```python
from build123d import *

# Parameters (mm, degrees)
SKETCH1_R               = 0.75
SKETCH1_R_2             = 1.5
BOSS_EXTRUDE1_DEPTH     = 3
CORTAR_EXTRUIR1_START   = -3
CROQUIS1_W              = 15
CROQUIS1_H              = 6.71890751
CORTAR_EXTRUIR1_DEPTH   = 3
CROQUIS2_W              = 30
CROQUIS2_H              = 3
SALIENTE_EXTRUIR1_DEPTH = 3


with BuildPart() as part:
    # Sketch1 → Boss-Extrude1 (new body)
    with BuildSketch(Plane.XY):
        Polygon((10, 0), (10, 3), (15, 3), (15, 0), (20, 0), (20, 3), (25, 3), (25, 0), (30, 0), (30, -26), (25, -26), (25, -29), (20, -29), (20, -26), (15, -26), (15, -29), (10, -29), (10, -26), (5, -26), (5, -29), (0, -29), (0, 0), align=None)
        with Locations((20.5, -5.5)):
            Circle(SKETCH1_R, mode=Mode.SUBTRACT)
        with Locations((26.995190528, -9.25)):
            Circle(SKETCH1_R, mode=Mode.SUBTRACT)
        with Locations((26.995190528, -16.75)):
            Circle(SKETCH1_R, mode=Mode.SUBTRACT)
        with Locations((20.5, -20.5)):
            Circle(SKETCH1_R, mode=Mode.SUBTRACT)
        with Locations((14.004809472, -16.75)):
            Circle(SKETCH1_R, mode=Mode.SUBTRACT)
        with Locations((14.004809472, -9.25)):
            Circle(SKETCH1_R, mode=Mode.SUBTRACT)
        with Locations((20.5, -13)):
            Circle(SKETCH1_R_2, mode=Mode.SUBTRACT)
    extrude(amount=BOSS_EXTRUDE1_DEPTH)

    # Croquis1 → Cortar-Extruir1 (cut)
    with BuildSketch(Plane.XY.offset(3).offset(CORTAR_EXTRUIR1_START)):
        with Locations((17.5, 3.359453755)):
            Rectangle(CROQUIS1_W, CROQUIS1_H)
    extrude(amount=CORTAR_EXTRUIR1_DEPTH, mode=Mode.SUBTRACT)

    # Croquis2 → Saliente-Extruir1 (add)
    with BuildSketch(Plane.XY.offset(3)):
        with Locations((15, 1.5)):
            Rectangle(CROQUIS2_W, CROQUIS2_H)
    extrude(amount=-SALIENTE_EXTRUIR1_DEPTH)


solid = part.part
```
Geometry check sheet. Reference: the model listing, model coordinates, mm. A direction names the side the tool comes from. Give positions to 0.01 mm unless a question says otherwise; leave off trailing zeros. Write each loop counter-clockwise with the first axis right and the second up, starting at its lowest first coordinate (ties: lowest second). Pieces come first, ordered by that corner, then holes. Notation, with made-up numbers: (89, 14.25) -> (134, 14.25) arc R16 ccw to (134, 27.25) -> close; hole circle Ø1 at (65.25, -13.75). An arc over 180 degrees is marked (long way). Use one line per item in the form item = value.
Item 1: Access from +Z, -Z, +X, -X, +Y, -Y to the whole of each face (thin tool, end or side, straight path). Record for faces 1 (the flat face through (20, -28, 1)), 2 (the flat face through (15, -13, 0)), 3 (the flat face through (28, -26, 1)).
Results list:
face_1 = +Z, -Z, -Y
face_2 = -Z, +X, -X, +Y, -Y
face_3 = +Z, -Z, +X, -Y
Item 2: Mould release check, pull along Y, two halves, no side actions. Record for faces 4 (the cylindrical face through (19.905, -20.956, 1.479)), 5 (the cylindrical face through (26.246, -9.217, 1.479)), 6 (the flat face through (5, -27, 1)), 7 (the flat face through (18, -26, 1)): released by +Y, released by -Y, zero draft, split by the parting line, or undercut.
Results list:
face_4 = undercut
face_5 = undercut
face_6 = zero draft
face_7 = released by -Y
Item 3: Sectioned sample at B-B on y = -20.5. Enter the section's corners in (x, z), plus the area to 3 significant figures.
Results list:
outline = (0, 0) -> (19.75, 0) -> (19.75, 3) -> (0, 3) -> close; (21.25, 0) -> (30, 0) -> (30, 3) -> (21.25, 3) -> close
area = 85.5 mm2
Item 4: Depth check by flat-ended pin: pin 1 Ø1.4 at (x, y) = (27, -16.75) entering from +Z; pin 2 Ø0.9 at (x, z) = (18.5, 2) entering from -Y; pin 3 Ø1.5 at (y, z) = (-27, 1.5) entering from +X. Enter the tip coordinate at first touch or a pass-through.
Results list:
pin_1 = through
pin_2 = -26
pin_3 = 25
Item 5: Sectioned sample at A-A on x = 20.5. Enter the section's corners in (y, z), plus the area to 3 significant figures.
Results list:
outline = (-29, 0) -> (-21.25, 0) -> (-21.25, 3) -> (-29, 3) -> close; (-19.75, 0) -> (-14.5, 0) -> (-14.5, 3) -> (-19.75, 3) -> close; (-11.5, 0) -> (-6.25, 0) -> (-6.25, 3) -> (-11.5, 3) -> close; (-4.75, 0) -> (3, 0) -> (3, 3) -> (-4.75, 3) -> close
area = 78.0 mm2
Item 6: Sectioned sample at D-D on y = -16.75. Enter the section's corners in (x, z).
Results list:
outline = (0, 0) -> (13.25, 0) -> (13.25, 3) -> (0, 3) -> close; (14.75, 0) -> (26.25, 0) -> (26.25, 3) -> (14.75, 3) -> close; (27.75, 0) -> (30, 0) -> (30, 3) -> (27.75, 3) -> close
Item 7: Scan lines: line 1 (X direction, y = -27, z = 0.25); line 2 (Y direction, x = 20.5, z = 1.1); line 3 (Y direction, x = 14.5, z = 0.3). Record each from-to range of solid material in increasing order.
Results list:
line_1 = 0 to 5, 10 to 15, 20 to 25
line_2 = -29 to -21.25, -19.75 to -14.5, -11.5 to -6.25, -4.75 to 3
line_3 = -29 to -17.31, -16.19 to -9.81, -8.69 to 3
Item 8: Sectioned sample at C-C on z = 0.9. Enter the section's corners in (x, y), plus the area to 3 significant figures.
Results list:
outline = (0, -29) -> (5, -29) -> (5, -26) -> (10, -26) -> (10, -29) -> (15, -29) -> (15, -26) -> (20, -26) -> (20, -29) -> (25, -29) -> (25, -26) -> (30, -26) -> (30, 3) -> (0, 3) -> close; hole circle Ø1.5 at (14, -16.75); hole circle Ø1.5 at (14, -9.25); hole circle Ø3 at (20.5, -13); hole circle Ø1.5 at (20.5, -20.5); hole circle Ø1.5 at (20.5, -5.5); hole circle Ø1.5 at (27, -16.75); hole circle Ø1.5 at (27, -9.25)
area = 897 mm2
